The model under review builds one solid part; all positions refer to its coordinate system, in mm. A direction names the side the tool comes from. Round coordinates to 2 decimals unless told otherwise and drop trailing zeros. Loops run counter-clockwise (first coordinate to the right, second up) from the corner with the lowest first, then second, coordinate; pieces in that order, holes last. Notation, with made-up numbers: (77.5, 80.5) -> (101.5, 80.5) arc R4 cw to (101.5, 87.5) -> close; hole circle Ø8 at (50.5, -20). An arc over 180 degrees is marked (long way). Return JSON: item names as keys, results as strings. Group by question number.
```python
from build123d import *

# Parameters (mm, degrees)
F1_DEPTH = 4
F2_W     = 5
F2_H     = 2.25
F2_W_2   = 8.75
F2_H_2   = 15
F2_H_3   = 21.35
F2_H_4   = 5
F3_DEPTH = 2


with BuildPart() as f1:
    # F0 (on Top) → F1 (new body)
    with BuildSketch(Plane.XY):
        with BuildLine():
            Line((48.35, 0), (3, 0))
            Line((3, 0), (3, -1.5))
            ThreePointArc((3, -1.5), (4.06066, -1.93934), (4.5, -3))
            ThreePointArc((4.5, -3), (3, -4.5), (1.5, -3))
            Line((1.5, -3), (0, -3))
            Line((0, -3), (0, -48.35))
            Line((0, -48.35), (1.5, -48.35))
            ThreePointArc((1.5, -48.35), (3, -46.85), (4.5, -48.35))
            ThreePointArc((4.5, -48.35), (4.06066, -49.41066), (3, -49.85))
            Line((3, -49.85), (3, -51.35))
            Line((3, -51.35), (48.35, -51.35))
            Line((48.35, -51.35), (48.35, -49.85))
            ThreePointArc((48.35, -49.85), (47.28934, -47.28934), (49.85, -48.35))
            Line((49.85, -48.35), (51.35, -48.35))
            Line((51.35, -48.35), (51.35, -3))
            Line((51.35, -3), (49.85, -3))
            ThreePointArc((49.85, -3), (47.28934, -4.06066), (48.35, -1.5))
            Line((48.35, -1.5), (48.35, 0))
        make_face()
        with BuildLine():
            Line((1.5, -48.35), (0, -48.35))
            Line((0, -48.35), (0, -51.35))
            Line((0, -51.35), (3, -51.35))
            Line((3, -51.35), (3, -49.85))
            ThreePointArc((3, -49.85), (1.93934, -49.41066), (1.5, -48.35))
        make_face()
        with BuildLine():
            Line((51.35, -51.35), (51.35, -48.35))
            Line((51.35, -48.35), (49.85, -48.35))
            ThreePointArc((49.85, -48.35), (49.41066, -49.41066), (48.35, -49.85))
            Line((48.35, -49.85), (48.35, -51.35))
            Line((48.35, -51.35), (51.35, -51.35))
        make_face()
        with BuildLine():
            Line((51.35, 0), (48.35, 0))
            Line((48.35, 0), (48.35, -1.5))
            ThreePointArc((48.35, -1.5), (49.41066, -1.93934), (49.85, -3))
            Line((49.85, -3), (51.35, -3))
            Line((51.35, -3), (51.35, 0))
        make_face()
        with BuildLine():
            Line((3, 0), (0, 0))
            Line((0, 0), (0, -3))
            Line((0, -3), (1.5, -3))
            ThreePointArc((1.5, -3), (1.93934, -1.93934), (3, -1.5))
            Line((3, -1.5), (3, 0))
        make_face()
    extrude(amount=F1_DEPTH)

    # F2 (on face) → F3 (cut)
    with BuildSketch(Plane.XY.offset(4)):
        with Locations((3.75, -9.875)):
            Rectangle(F2_W, F2_H)
        with Locations((4.375, -27)):
            Rectangle(F2_W_2, F2_H_2)
        with BuildLine():
            Line((16, -37.35), (13.7, -37.35))
            ThreePointArc((13.7, -37.35), (14.373654, -38.976346), (16, -39.65))
            Line((16, -39.65), (16, -37.35))
        make_face()
        with BuildLine():
            ThreePointArc((18.3, -37.35), (16, -35.05), (13.7, -37.35))
            Line((13.7, -37.35), (16, -37.35))
            Line((16, -37.35), (16, -39.65))
            ThreePointArc((16, -39.65), (17.626346, -38.976346), (18.3, -37.35))
        make_face()
        with BuildLine():
            ThreePointArc((37.65, -37.35), (33.723654, -35.723654), (35.35, -39.65))
            Line((35.35, -39.65), (35.35, -37.35))
            Line((35.35, -37.35), (37.65, -37.35))
        make_face()
        with BuildLine():
            Line((35.35, -37.35), (35.35, -39.65))
            ThreePointArc((35.35, -39.65), (36.976346, -38.976346), (37.65, -37.35))
            Line((37.65, -37.35), (35.35, -37.35))
        make_face()
        with Locations((46.975, -26.675)):
            Rectangle(F2_W_2, F2_H_3)
        with Locations((46.975, -39.85)):
            Rectangle(F2_W_2, F2_H_4)
        with Locations((10, -3.025)):
            Rectangle(F2_W, F2_H)
    extrude(amount=-F3_DEPTH, mode=Mode.SUBTRACT)


solid = f1.part
```
1. Tool access review of faces 5 (the face through (47, -29, 2)), 6 (the face through (0, -25.3, 1.5)), 7 (the face through (8.75, -27, 3)), 8 (the face through (10, -4.15, 3)), 9 (the face through (25, -25, 4)): name each direction out of +Z, -Z, +X, -X, +Y, -Y from which nothing blocks a thin tool from reaching the whole face with its end or side.
2. Draft analysis for pull direction X (two halves, no side actions). For faces 1 (the face through (51.35, -26, 1.5)), 2 (the face through (35, -37, 2)), 3 (the face through (4, -8.75, 3)), 4 (the face through (4, -34.5, 3)), state which applies: pulls with the +X half, pulls with the -X half, needs draft (parallel to the pull), parting line crosses it, or undercut.
3. Wall thickness on line 1 (Y direction, x = 48.35, z = 1.7); line 2 (Y direction, x = 48.35, z = 3.15); line 3 (X direction, y = -48.35, z = 3.1): over which ranges is each line inside the solid? List them lowest first.
4. For P1, Ø2.5, axis at x = 48.35, y = -3, coming from the -Z side; P2, Ø1.8, axis at x = 3.5, y = -10, coming from the +Z side; P3, Ø1.6, axis at y = -28, z = 3.5, coming from the -X side; P4, Ø1, axis at y = -30, z = 3.5, coming from the +X side, all flat-tipped, find the tip position at first contact; note any pin that passes through.
5. We need section A-A, the plane y = -20.5. Write out the cut boundary in (x, z).
6. We need section B-B, the plane x = 47.5. Write out the cut boundary in (y, z).
Check sheet entries:
{
 "1": {"face 5": "+Z, +X", "face 6": "+Z, -Z, -X, +Y, -Y", "face 7": "+Z, -X", "face 8": "+Z", "face 9": "+Z, +X, -X, +Y, -Y"},
 "2": {"face 1": "pulls with the +X half", "face 2": "undercut", "face 3": "undercut", "face 4": "needs draft"},
 "3": {"line 1": "y = -51.35 to -49.85, -46.85 to -4.5, -1.5 to 0", "line 2": "y = -51.35 to -49.85, -46.85 to -42.35, -16 to -4.5, -1.5 to 0", "line 3": "x = 0 to 1.5, 4.5 to 46.85, 49.85 to 51.35"},
 "4": {"P1": "passes through", "P2": "stops at z = 2", "P3": "stops at x = 8.75", "P4": "stops at x = 42.6"},
 "5": {"outline": "(0, 0) -> (51.35, 0) -> (51.35, 2) -> (42.6, 2) -> (42.6, 4) -> (8.75, 4) -> (8.75, 2) -> (0, 2) -> close"},
 "6": {"outline": "(-51.35, 0) -> (-49.59, 0) -> (-49.59, 4) -> (-51.35, 4) -> close; (-47.11, 0) -> (-4.24, 0) -> (-4.24, 4) -> (-16, 4) -> (-16, 2) -> (-42.35, 2) -> (-42.35, 4) -> (-47.11, 4) -> close; (-1.76, 0) -> (0, 0) -> (0, 4) -> (-1.76, 4) -> close"}
}
